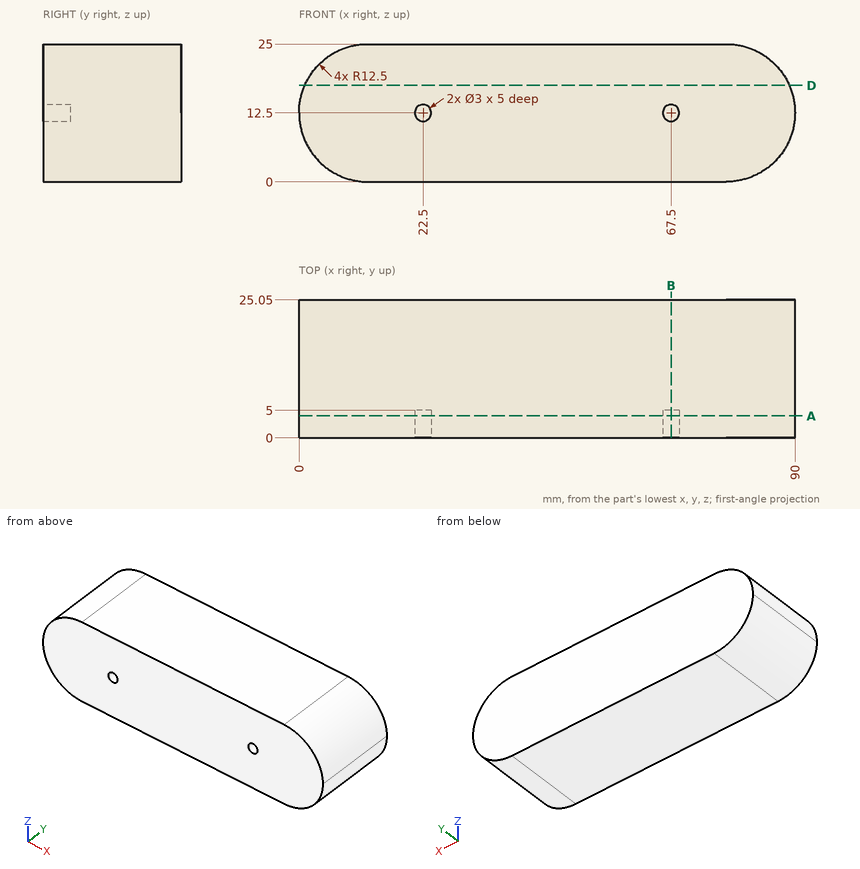
Input: dimensioned drawing with shaded views. Units: mm. Origin: part minimum x, y, z. Coordinates: 2 decimals unless noted, no trailing zeros. Loops run counter-clockwise (first coordinate to the right, second up) from the corner with the lowest first, then second, coordinate; pieces in that order, holes last. Notation, with made-up numbers: M 61,82 L 73,82 A14 ccw 73,97 Z; hole C 89.5,36 d7. An arc over 180 degrees is marked long. Use a Markdown table: item, result. Add a question column.
Q1. First-contact query: pin 1 (3 mm diameter, centred on y = 8.5, z = 17.5, fed in from +X); pin 2 (2.5 mm diameter, centred on x = 67.5, z = 12.5, fed in from -Y). Flat tips, straight axial feed; report the tip coordinate or a pass-through.
Q2. Section query D-D, the plane z = 17.5. Return loops of the section in (x, y), and give its area (3 significant figures).
Q3. Material intervals for L1, parallel to X at y = 3.75, z = 12.5; L2, parallel to X at y = 2.25, z = 19; L3, parallel to X at y = 17.75, z = 14.75, sorted ascending.
Q4. Section query B-B, the plane x = 67.5. Return loops of the section in (y, z).
Q5. Section query A-A, the plane y = 4. State how many separate pieces and enclosed holes the cut face has, and give its area (3 significant figures).
Result:
| question | item | result |
|---|---|---|
| 1 | pin 1 | stops at x = 89.5 |
| 1 | pin 2 | stops at y = 5 |
| 2 | outline | M 1.04,0 L 88.96,0 L 88.96,25.05 L 1.04,25.05 Z |
| 2 | area | 2,200 mm2 |
| 3 | L1 | x = 0 to 21, 24 to 66, 69 to 90 |
| 3 | L2 | x = 1.82 to 88.18 |
| 3 | L3 | x = 0.2 to 89.8 |
| 4 | outline | M 0,0 L 25.05,0 L 25.05,25 L 0,25 L 0,14 L 5,14 L 5,11 L 0,11 Z |
| 5 | separate pieces | 1 |
| 5 | enclosed holes | 2 |
| 5 | area | 2,100 mm2 |
